Job drawing, mm, ordinate dimensions from the low corner. One solid piece. Coordinates: 2 decimals unless noted, no trailing zeros. Loops run counter-clockwise (first coordinate to the right, second up) from the corner with the lowest first, then second, coordinate; pieces in that order, holes last. Notation, with made-up numbers: M 2,-30.75 L 40,-30.75 A7 cw 40,-18.75 Z; hole C 18,-31.5 d9. An arc over 180 degrees is marked long. Answer as a JSON object with one key per item and string values. Group by question number.
1. Drop flat-ended pins along their axis: pin 1 Ø1.5 at (y, z) = (57, 2) entering from +X; pin 2 Ø0.9 at (x, z) = (15, 1) entering from +Y; pin 3 Ø0.9 at (y, z) = (44, 1) entering from -X. Give the stop position or say it passes through.
2. Saw through at C-C on x = 123.5. Write the cut outline in (y, z), then the cut area to 3 significant figures.
3. Drill centre lines: L1, parallel to X at y = 50.5, z = 2.75; L2, parallel to Y at x = 86, z = 1.9. Where is each one in solid material? Low to high.
4. Saw through at B-B on y = 15.5. Write the cut outline in (x, z).
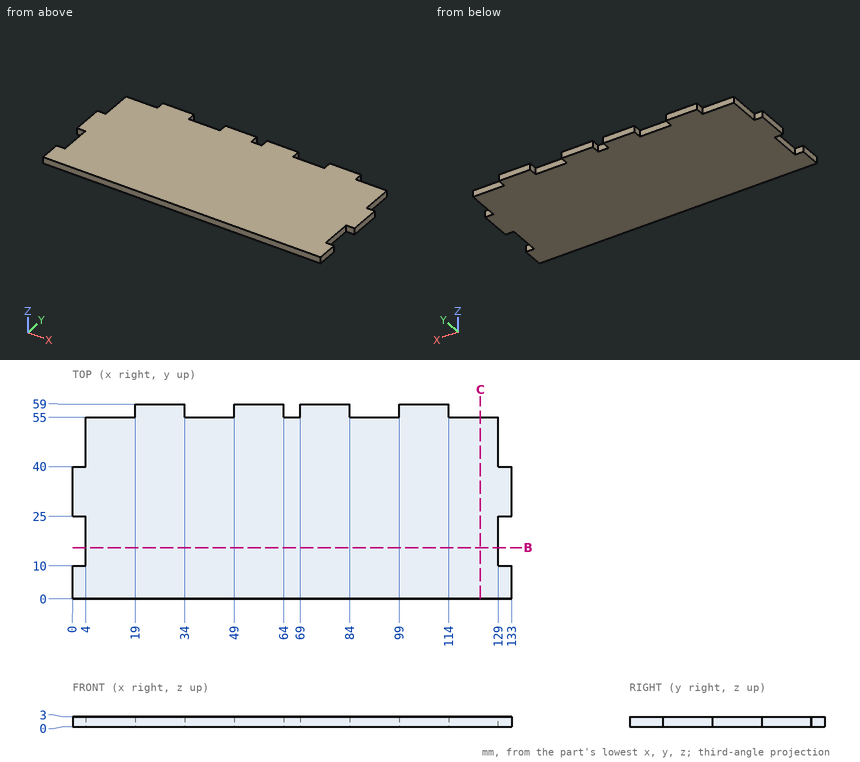
Outcome:
{
 "1": {"pin 1": "stops at x = 114", "pin 2": "stops at y = 55", "pin 3": "stops at x = 4"},
 "2": {"outline": "M 0,0 L 55,0 L 55,3 L 0,3 Z", "area": "165 mm²"},
 "3": {"L1": "x = 4 to 129", "L2": "y = 0 to 55"},
 "4": {"outline": "M 4,0 L 129,0 L 129,3 L 4,3 Z"}
}
